Part model, mm, in its own coordinate system. A direction names the side the tool comes from. Coordinates: 2 decimals unless noted, no trailing zeros. Loops run counter-clockwise (first coordinate to the right, second up) from the corner with the lowest first, then second, coordinate; pieces in that order, holes last.
```python
from build123d import *

# Parameters (mm, degrees)
EXTRUDE_1_DEPTH       = 10
FILLET_1_R            = 2
HOLE_WIZARD_M51_D     = 5.5
HOLE_WIZARD_M51_DEPTH = 5
M5X0_81_D             = 4.2
M5X0_82_D             = 4.2
M5X0_82_DEPTH         = 10
M5X0_82_TIP           = 1.2618073


with BuildPart() as part:
    # Эскиз1 → Бобышка-Вытянуть1 (new body)
    with BuildSketch(Plane.XY):
        with BuildLine():
            Line((32, -3), (19.773719933, -3))
            ThreePointArc((19.773719933, -3), (-19.993649721, 0.503955172), (19.899748742, 2))
            Line((19.899748742, 2), (32, 2))
            Line((32, 2), (32, 7))
            Line((32, 7), (21.9089023, 7))
            ThreePointArc((21.9089023, 7), (-3.54226249, 22.725588583), (-23, 0))
            Line((-23, 0), (-23, -28))
            Line((-23, -28), (32, -28))
            Line((32, -28), (32, -3))
        make_face()
    extrude(amount=EXTRUDE_1_DEPTH)

    # Скругление1
    fillet_1_edges = [part.edges().sort_by_distance(p)[0] for p in [
        (21.9089023, 7, 5),
        (32, 7, 5),
        (32, 2, 5),
        (19.899748742, 2, 5),
        (19.773719933, -3, 5),
        (32, -3, 5),
    ]]
    fillet(fillet_1_edges, radius=FILLET_1_R)

    # Отверстие с зазором M51
    with Locations(Plane(origin=(0, 7, 0), x_dir=(1, 0, 0), z_dir=(0, 1, 0))):
        with Locations((26.95445115, -5)):
            Hole(HOLE_WIZARD_M51_D / 2, depth=HOLE_WIZARD_M51_DEPTH)

    # Отверстие обработанное метчиком M5x0.81 (through all)
    with Locations(Plane(origin=(0, -3, 0), x_dir=(1, 0, 0), z_dir=(0, 1, 0))):
        with Locations((26.95445115, -5)):
            Hole(M5X0_81_D / 2)

    # Отверстие обработанное метчиком M5x0.82
    with Locations(Plane(origin=(0, -28, 0), x_dir=(-1, 0, 0), z_dir=(0, -1, 0))):
        with Locations((15, -5)):
            Hole(M5X0_82_D / 2, depth=M5X0_82_DEPTH)
            with Locations((0, 0, -(M5X0_82_DEPTH + M5X0_82_TIP / 2))):  # 118° drill point
                Cone(0, M5X0_82_D / 2, M5X0_82_TIP, mode=Mode.SUBTRACT)


solid = part.part
```
Q1. Tool access for faces 1 (the conical face through (-15.35, -16.96, 4.89)), 2 (the cylindrical face through (31.4, 2.57, 5.07)), 3 (the cylindrical face through (20.2, -3.42, 5.07)): list every direction of +Z, -Z, +X, -X, +Y, -Y with a clear straight run to the whole face (end or side of a thin tool).
Q2. Saw through at D-D (x = 28). List the corners of the cut face in (y, z), plus the area to 3 significant figures.
Q3. Probe line 1 (Z direction, x = -15, y = -22); line 2 (Y direction, x = 0, z = 4); line 3 (Y direction, x = 12.5, z = 2.5). List the from-to ranges inside material, lowest first.
Q4. Saw through at A-A (x = 0). List the corners of the cut face in (y, z), plus the area to 3 significant figures.
Q5. Saw through at B-B (y = -10). List the corners of the cut face in (x, z).
Q6. Mould opens along Z. For faces 4 (the flat face through (24, 7, 5)), 5 (the cylindrical face through (24.414, 4.465, 6.053)), 6 (the cylindrical face through (-15.46, -22.93, 7.05)), 7 (the flat face through (10, -19, 0)) say: released by +Z, released by -Z, zero draft, split by the parting line, or undercut.
Q7. Saw through at C-C (y = 11). List the corners of the cut face in (x, z), plus the area to 3 significant figures.
Q8. Drop flat-ended pins along their axis: P1, Ø3.5, axis at x = 28, z = 3.5, coming from the +Y side; P2, Ø4, axis at y = 3, z = 3, coming from the -X side; P3, Ø4, axis at x = -15, z = 5, coming from the -Y side. Give the stop position or say it passes through.
Checked values:
1. face 1: -Y
1. face 2: +Z, -Z, +X
1. face 3: +Z, -Z
2. outline: (-28, 0) - (-3, 0) - (-3, 3.18) - (-28, 3.18) - close; (-28, 6.82) - (-3, 6.82) - (-3, 10) - (-28, 10) - close; (2, 0) - (7, 0) - (7, 2.46) - (2, 2.46) - close; (2, 7.54) - (7, 7.54) - (7, 10) - (2, 10) - close
2. area: 184 mm2
3. line 1: z = 0 to 2.9, 7.1 to 10
3. line 2: y = -28 to -20, 20 to 23
3. line 3: y = -28 to -15.61, 15.61 to 19.31
4. outline: (-28, 0) - (-20, 0) - (-20, 10) - (-28, 10) - close; (20, 0) - (23, 0) - (23, 10) - (20, 10) - close
4. area: 110 mm2
5. outline: (-23, 0) - (-17.32, 0) - (-17.32, 10) - (-23, 10) - close; (17.32, 0) - (32, 0) - (32, 10) - (17.32, 10) - close; hole circle Ø4.2 at (26.95, 5)
6. face 4: zero draft
6. face 5: undercut
6. face 6: undercut
6. face 7: released by -Z
7. outline: (-20.2, 0) - (-16.7, 0) - (-16.7, 10) - (-20.2, 10) - close; (16.7, 0) - (20.2, 0) - (20.2, 10) - (16.7, 10) - close
7. area: 69.9 mm2
8. P1: stops at y = 7
8. P2: stops at x = -22.98
8. P3: stops at y = -17.94
